Part model, mm, in its own coordinate system. Face numbers are marked on the shaded views. Round coordinates to 2 decimals unless told otherwise and drop trailing zeros. Loops run counter-clockwise (first coordinate to the right, second up) from the corner with the lowest first, then second, coordinate; pieces in that order, holes last. Notation, with made-up numbers: (27.5, 24) -> (79.5, 24) arc R18 ccw to (79.5, 42) -> close; hole circle Ø8 at (24.25, -38). An arc over 180 degrees is marked (long way). Answer as a JSON object with one key per item and string values. Group by question number.
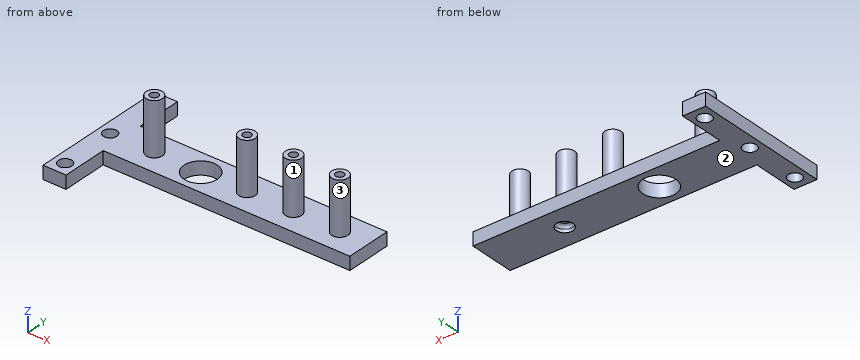
Autodesk Inventor part; units mm, degrees
ref_plane "YZ Plane" through (0, 0, 0) normal (1, 0, 0) x (0, 1, 0)
ref_plane "XZ Plane" through (0, 0, 0) normal (0, 1, 0) x (-1, 0, 0)
ref_plane "XY Plane" through (0, 0, 0) normal (0, 0, 1) x (1, 0, 0)
sketch "Sketch1" plane through (0, 0, 0) normal (0, 0, 1) x (1, 0, 0)
  line L0 (0, 0) -> (42, 0)
  line L1 (42, 0) -> (42, 14)
  line L2 (42, 14) -> (0, 14)
  line L3 (0, 14) -> (0, 0)
  dimension "d0" = 42
  dimension "d1" = 14
extrude "Extrusion1" add sketch "Sketch1" along normal blind 4
sketch "Sketch2" plane through (0, 0, 4) normal (0, 0, 1) x (1, 0, 0)
  circle A0 centre (21, 7) radius 2.55
  line L0 (42, 14) -> (0, 14)
  line L1 (0, 14) -> (0, 0)
  circle A1 centre (6.9, 7) radius 2.5
  circle A2 centre (35.1, 7) radius 2.5
  dimension "d35" = 0
  dimension "d4" = 5.1
  dimension "d5" = 42
  dimension "d6" = 14
  dimension "d7" = 7
  dimension "d8" = 21
  dimension "d9" = 5
  dimension "d10" = 5
  dimension "d11" = 14.1
  dimension "d12" = 14.1
extrude "Extrusion2" add sketch "Sketch2" along normal blind 16 contours A1 | A2
extrude "Extrusion3" cut sketch "Sketch2" against normal blind 4 contours A0
sketch "Sketch3" plane through (6.9, 7, 20) normal (0, 0, 1) x (1, 0, 0)
  circle A0 centre (0, 0) radius 1.25
  circle A1 centre (28.2, 0) radius 2.5
  circle A2 centre (28.2, 0) radius 1.25
  point P0 (-6.9, -7)
  dimension "d19" = 2.5
  dimension "d20" = 2.5
extrude "Extrusion4" cut sketch "Sketch3" against normal blind 3 contours A0 | A2
sketch "Sketch4" plane through (0, 0, 0) normal (0, 0, -1) x (-1, 0, 0)
  circle A0 centre (-21, 7) radius 2.55
  circle A1 centre (-49.8, 7) radius 2.55
  point P0 (0, 0)
  dimension "d23" = 5.1
  dimension "d24" = 28.8
sketch "Sketch5" plane through (42, 0, 0) normal (1, 0, 0) x (0, 0, -1)
  line L0 (0, 0) -> (-4, 0)
  line L1 (-4, 14) -> (0, 14)
  line L2 (0, 14) -> (0, 0)
  line L3 (0, 0) -> (-4, 0)
  line L4 (-4, 0) -> (-4, 14)
extrude "Extrusion5" add sketch "Sketch5" along normal blind 30
extrude "Extrusion6" cut sketch "Sketch4" against normal blind 2 contours A1
sketch "Sketch6" plane through (0, 0, 0) normal (0, 0, -1) x (-1, 0, 0)
  circle A0 centre (-21, 7) radius 2.55
  circle A1 centre (-21, 7) radius 5.05
  point P0 (0, 0)
  dimension "d29" = 10.1
extrude "Extrusion7" cut sketch "Sketch6" against normal through all
sketch "Sketch7" plane through (0, 0, 4) normal (0, 0, 1) x (1, 0, 0)
  circle A0 centre (35.1, 7) radius 2.5
  circle A1 centre (49.2, 7) radius 2.5
  point P0 (0, 0)
  dimension "d32" = 5
  dimension "d33" = 14.1
extrude "Extrusion8" add sketch "Sketch7" along normal blind 16 contours A1
fillet "Fillet3" radius 1 1 edges at (52.35, 7, 2)
sketch "Sketch8" plane through (49.2, 7, 20) normal (0, 0, 1) x (1, 0, 0)
  circle A0 centre (0, 0) radius 1.25
  point P0 (-49.2, -7)
  dimension "d37" = 2.5
extrude "Extrusion9" cut sketch "Sketch8" against normal blind 3
pattern_linear "Rectangular Pattern1" count 2 spacing 14.1 along (1, 0, 0) of "Extrusion8", "Extrusion9"
sketch "Sketch9" plane through (0, 0, 0) normal (-1, 0, 0) x (0, 0, 1)
  line L0 (4, 14) -> (4, 0)
  line L1 (0, 0) -> (4, 0)
  line L2 (4, 0) -> (4, 14)
  line L3 (4, 14) -> (0, 14)
  line L4 (0, 14) -> (0, 0)
extrude "Extrusion10" add sketch "Sketch9" along normal blind 10
sketch "Sketch10" plane through (72, 0, 0) normal (0, -1, 0) x (1, 0, 0)
  line L0 (0, 4) -> (-82, 4)
  line L1 (-82, 0) -> (0, 0)
  line L2 (-82, 4) -> (-75, 4)
  line L3 (-75, 4) -> (-75, 0)
  line L4 (-75, 0) -> (-82, 0)
  line L5 (-82, 0) -> (-82, 4)
  point P0 (-72, 0)
  dimension "d46" = 7
extrude "Extrusion11" add sketch "Sketch10" along normal blind 14
sketch "Sketch11" plane through (72, 14, 4) normal (0, 1, 0) x (1, 0, 0)
  line L0 (-82, 0) -> (-82, 4)
  line L1 (-82, 4) -> (-75, 4)
  line L2 (-82, 0) -> (-75, 0)
  line L3 (-75, 0) -> (-75, 4)
  line L4 (-75, 4) -> (-82, 4)
  line L5 (-82, 4) -> (-82, 0)
  point P0 (-72, 4)
  dimension "d49" = 7
extrude "Extrusion12" add sketch "Sketch11" along normal blind 14
sketch "Sketch12" plane through (0, 0, 4) normal (0, 0, 1) x (1, 0, 0)
  circle A0 centre (-6.5, 24) radius 2.05
  line L0 (-3, 14) -> (-3, 28)
  line L1 (-10, 28) -> (-3, 28)
  circle A1 centre (-6.5, 7) radius 2.05
  circle A2 centre (-6.5, -10) radius 2.05
  point P0 (0, 0)
  dimension "d52" = 4.1
  dimension "d53" = 3.5
  dimension "d54" = 4
  dimension "d57" = 17
extrude "Extrusion13" cut sketch "Sketch12" against normal through all
equation "\"d7\" = 0.5 * d6"
equation "\"d8\" = 0.5 * d5"
properties part number "Kroller Holder"
Item 1: Band-saw the part on C-C, the plane z = 8.75. List the corners of the cut face in (x, y), plus the area to 3 significant figures.
Item 2: Band-saw the part on B-B, the plane y = 24. List the corners of the cut face in (x, z).
Item 3: Two-plate mould, pull along X, no slides. Class the marked faces 1, 2 and 3: pulls with the +X half, pulls with the -X half, needs draft (parallel to the pull), parting line crosses it, or undercut.
Item 4: Band-saw the part on A-A, the plane x = 6.9. List the corners of the cut face in (y, z), plus the area to 4 significant figures.
Item 5: Drop flat-ended pins along their axis: pin 1 Ø8 at (x, z) = (51, 10) entering from -Y; pin 2 Ø4.5 at (y, z) = (18, 1.5) entering from +X; pin 3 Ø11.5 at (x, y) = (21, 7) entering from +Z. Give the stop position or say it passes through.
Item 6: Drill centre lines: line 1 (Y direction, x = -6.5, z = 1.05); line 2 (Y direction, x = 49.2, z = 18.4); line 3 (Y direction, x = 21, z = 1.55). Where is each one in solid material? Low to high.
Item 7: Band-saw the part on D-D, the plane y = 10.5. List the corners of the cut face in (x, z), plus the area to 3 significant figures.
Entries:
{
 "1": {"outline": "circle Ø5 at (6.9, 7); circle Ø5 at (35.1, 7); circle Ø5 at (49.2, 7); circle Ø5 at (63.3, 7)", "area": "78.5 mm²"},
 "2": {"outline": "(-10, 0) -> (-8.55, 0) -> (-8.55, 4) -> (-10, 4) -> close; (-4.45, 0) -> (-3, 0) -> (-3, 4) -> (-4.45, 4) -> close"},
 "3": {"face 1": "undercut", "face 2": "needs draft", "face 3": "undercut"},
 "4": {"outline": "(0, 0) -> (14, 0) -> (14, 4) -> (9.5, 4) -> (9.5, 20) -> (8.25, 20) -> (8.25, 17) -> (5.75, 17) -> (5.75, 20) -> (4.5, 20) -> (4.5, 4) -> (0, 4) -> close", "area": "128.5 mm²"},
 "5": {"pin 1": "y = 4.5", "pin 2": "x = -3", "pin 3": "z = 4"},
 "6": {"line 1": "-14 to -12.05, -7.95 to 4.95, 9.05 to 21.95, 26.05 to 28", "line 2": "4.5 to 5.75, 8.25 to 9.5", "line 3": "0 to 1.95, 12.05 to 14"},
 "7": {"outline": "(-10, 0) -> (17.36, 0) -> (17.36, 4) -> (-10, 4) -> close; (24.64, 0) -> (72, 0) -> (72, 4) -> (24.64, 4) -> close", "area": "299 mm²"}
}
